Print and shaded views of the part. All mm, measured from the part's lowest x, y and z. Round coordinates to 2 decimals unless told otherwise and drop trailing zeros. Write each loop counter-clockwise with the first axis right and the second up, starting at its lowest first coordinate (ties: lowest second). Pieces come first, ordered by that corner, then holes. Notation, with made-up numbers: (-11, -9) - (-6, -9) arc R5 ccw to (-6, -1) - close; hole circle Ø7 at (82.5, 3.25). An arc over 180 degrees is marked (long way). Answer as a JSON object with one key per item and string values. Group by question number.
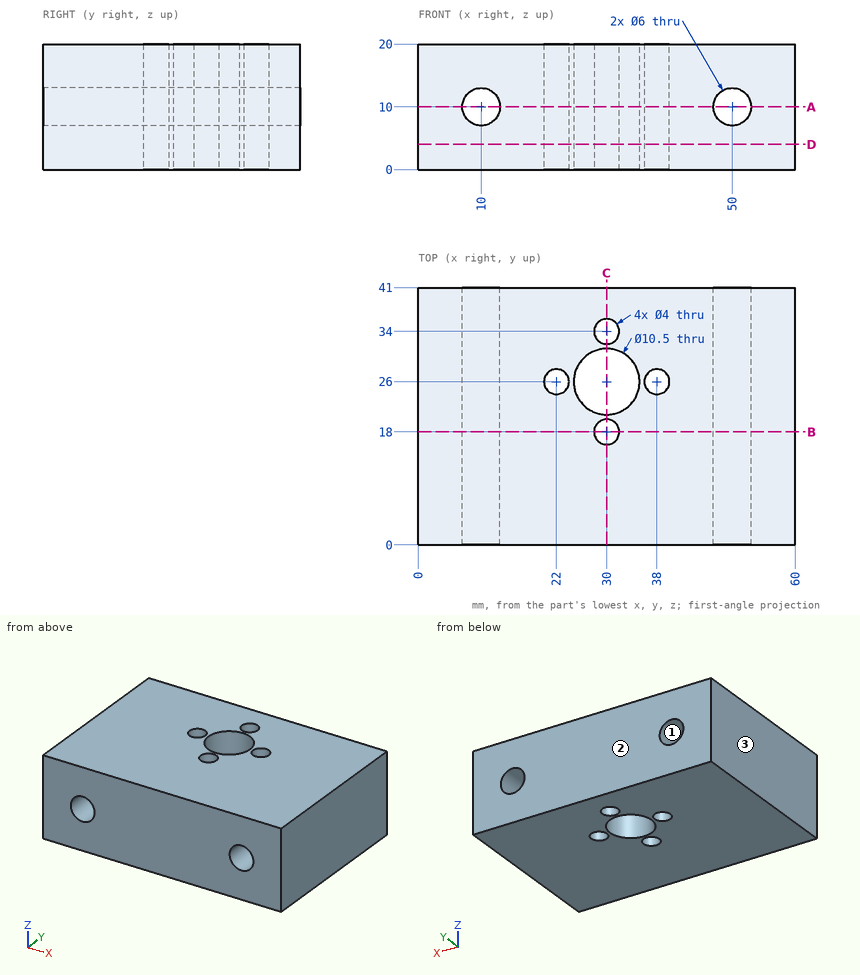
(1) Slice it at B-B (y = 18). Write the cut outline in (x, z), then the cut area to 3 significant figures.
(2) Pull direction X, two halves, no side cores. Call the marked faces 1, 2 and 3: pulls with the +X half, pulls with the -X half, needs draft (parallel to the pull), parting line crosses it, or undercut.
(3) Slice it at C-C (x = 30). Write the cut outline in (y, z), then the cut area to 3 significant figures.
(4) Flat gauge pin, fed straight in: pin 1 (2 mm diameter, centred on x = 32.5, y = 23.5, fed in from +Z). Where does the tip first touch, or does it go through?
(5) Slice it at A-A (z = 10). Write the cut outline in (x, y), then the cut area to 3 significant figures.
(6) Drill centre lines: line 1 (Y direction, x = 30, z = 6.25); line 2 (X direction, y = 6, z = 12.25); line 3 (X direction, y = 25, z = 5.25). Where is each one in solid material? Low to high. Write a range as from..to.
(7) Slice it at D-D (z = 4). Write the cut outline in (x, y).
Answer:
{
 "1": {"outline": "(0, 0) - (28, 0) - (28, 20) - (0, 20) - close; (32, 0) - (60, 0) - (60, 20) - (32, 20) - close; hole circle Ø6 at (10, 10); hole circle Ø6 at (50, 10)", "area": "1,060 mm²"},
 "2": {"face 1": "undercut", "face 2": "needs draft", "face 3": "pulls with the -X half"},
 "3": {"outline": "(0, 0) - (16, 0) - (16, 20) - (0, 20) - close; (20, 0) - (20.75, 0) - (20.75, 20) - (20, 20) - close; (31.25, 0) - (32, 0) - (32, 20) - (31.25, 20) - close; (36, 0) - (41, 0) - (41, 20) - (36, 20) - close", "area": "450 mm²"},
 "4": {"pin 1": "through"},
 "5": {"outline": "(0, 0) - (7, 0) - (7, 41) - (0, 41) - close; (13, 0) - (47, 0) - (47, 41) - (13, 41) - close; (53, 0) - (60, 0) - (60, 41) - (53, 41) - close; hole circle Ø4 at (22, 26); hole circle Ø10.5 at (30, 26); hole circle Ø4 at (30, 18); hole circle Ø4 at (30, 34); hole circle Ø4 at (38, 26)", "area": "1,830 mm²"},
 "6": {"line 1": "0..16, 20..20.75, 31.25..32, 36..41", "line 2": "0..8.02, 11.98..48.02, 51.98..60", "line 3": "0..20.27, 23.73..24.85, 35.15..36.27, 39.73..60"},
 "7": {"outline": "(0, 0) - (60, 0) - (60, 41) - (0, 41) - close; hole circle Ø4 at (22, 26); hole circle Ø10.5 at (30, 26); hole circle Ø4 at (30, 18); hole circle Ø4 at (30, 34); hole circle Ø4 at (38, 26)"}
}
